from build123d import *

# Parameters (mm, degrees)
SKETCH1_R           = 16.15
BOSS_EXTRUDE1_DEPTH = 5.2
FILLET1_R           = 20
CHAMFER1_SIZE       = 1
SKETCH2_R           = 19.025242353
SKETCH2_R_2         = 14
BOSS_EXTRUDE2_DEPTH = 0.6
SKETCH4_R           = 18.71529055
SKETCH4_R_2         = 14
BOSS_EXTRUDE3_DEPTH = 1
CHAMFER2_SIZE       = 1


with BuildPart() as part:
    # Sketch1 → Boss-Extrude1 (new body)
    with BuildSketch(Plane(origin=(0, 0, 0), x_dir=(1, 0, 0), z_dir=(0, 1, 0))):
        with BuildLine():
            Line((50.6952797, -21), (63.625, -21))
            ThreePointArc((63.625, -21), (84.625, 0), (63.625, 21))
            Line((63.625, 21), (50.6952797, 21))
            ThreePointArc((50.6952797, 21), (44.646090821, 13.026866227), (35.106613419, 10))
            Line((35.106613419, 10), (-35.106613419, 10))
            ThreePointArc((-35.106613419, 10), (-44.646090821, 13.026866227), (-50.6952797, 21))
            Line((-50.6952797, 21), (-63.625, 21))
            ThreePointArc((-63.625, 21), (-84.625, 0), (-63.625, -21))
            Line((-63.625, -21), (-50.6952797, -21))
            ThreePointArc((-50.6952797, -21), (-44.646090821, -13.026866227), (-35.106613419, -10))
            Line((-35.106613419, -10), (35.106613419, -10))
            ThreePointArc((35.106613419, -10), (44.646090821, -13.026866227), (50.6952797, -21))
        make_face()
        with Locations((-63.625, 0)):
            Circle(SKETCH1_R, mode=Mode.SUBTRACT)
        with Locations((63.625, 0)):
            Circle(SKETCH1_R, mode=Mode.SUBTRACT)
    extrude(amount=BOSS_EXTRUDE1_DEPTH)

    # Fillet1
    fillet1_edges = [part.edges().sort_by_distance(p)[0] for p in [
        (-50.6952797, 2.6, 21),
        (-50.6952797, 2.6, -21),
        (50.6952797, 2.6, -21),
        (50.6952797, 2.6, 21),
    ]]
    fillet(fillet1_edges, radius=FILLET1_R)

    # Chamfer1
    chamfer1_edges = [part.edges().sort_by_distance(p)[0] for p in [
        (62.433003391, 5.2, 21),
        (84.625, 5.2, 0),
        (62.433003391, 5.2, -21),
        (41.52534742, 5.2, -11.295776268),
        (0, 5.2, -10),
        (41.52534742, 5.2, 11.295776268),
        (-41.52534742, 5.2, -11.295776268),
        (-62.433003391, 5.2, -21),
        (-62.433003391, 5.2, 21),
        (-53.482236449, 5.2, 19.433705079),
        (-53.482236449, 5.2, -19.433705079),
        (-84.625, 5.2, 0),
        (53.482236449, 5.2, -19.433705079),
        (53.482236449, 5.2, 19.433705079),
        (-41.52534742, 5.2, 11.295776268),
        (0, 5.2, 10),
        (47.475, 5.2, 0),
    ]]
    chamfer(chamfer1_edges, length=CHAMFER1_SIZE)

    # Sketch2 → Boss-Extrude2 (add)
    with BuildSketch(Plane.XZ):
        with Locations((63.625, 0)):
            Circle(SKETCH2_R)
        with Locations((63.625, 0)):
            Circle(SKETCH2_R_2, mode=Mode.SUBTRACT)
    extrude(amount=-BOSS_EXTRUDE2_DEPTH)

    # Sketch4 → Boss-Extrude3 (add)
    with BuildSketch(Plane(origin=(0, 5.2, 0), x_dir=(1, 0, 0), z_dir=(0, 1, 0))):
        with Locations((-63.625, 0)):
            Circle(SKETCH4_R)
        with Locations((-63.625, 0)):
            Circle(SKETCH4_R_2, mode=Mode.SUBTRACT)
    extrude(amount=-BOSS_EXTRUDE3_DEPTH)

    # Chamfer2
    chamfer2_edges = [part.edges().sort_by_distance(p)[0] for p in [
        (-79.775, 0, 0),
    ]]
    chamfer(chamfer2_edges, length=CHAMFER2_SIZE)


solid = part.part
Geometry: final body of the model. Coordinates: model frame, mm. A direction names the side the tool comes from. Give positions to 0.01 mm unless a question says otherwise; leave off trailing zeros. Write each loop counter-clockwise with the first axis right and the second up, starting at its lowest first coordinate (ties: lowest second). Pieces come first, ordered by that corner, then holes.
(1) Mould query, pull axis Z, two halves, no side actions, for faces 1 (the conical face through (-83.78, 5.04, -0.44)), 2 (the cylindrical face through (47.49, 2.37, -0.71)), 3 (the flat face through (0, 2, -10)), 4 (the flat face through (-76, 4.2, -7)). Classes: released by +Z, released by -Z, zero draft, split by the parting line, or undercut.
(2) Access query for faces 5 (the cylindrical face through (-53.4, 2.1, -19.4)), 6 (the cylindrical face through (-79.76, 2.58, -0.71)), 7 (the cylindrical face through (-53.4, 2.1, 19.4)), 8 (the flat face through (63.5, 0.6, 14.4)), 9 (the conical face through (83.78, 5.04, 0.44)). Directions: +Z, -Z, +X, -X, +Y, -Y. A direction counts if a zero-diameter tool reaches every point of the face in a straight line with its end or side. Return the directions, or none.
(3) Cut plane B-B, the plane y = 2.15. Give the number of separate pieces and of enclosed holes in the cut face, then the cut area to 3 significant figures.
(4) Ray query, line 1 (X direction, y = 1.35, z = 0) (3 decimals); line 2 (X direction, y = 3, z = 15); line 3 (X direction, y = 4.55, z = 0) (3 decimals). Return the intervals inside material, ascending.
(5) Cut plane A-A, the plane z = 0. Return loops of the section in (x, y) (3 decimals), then the cut area to 3 significant figures.
Values follow:
1. face 1: split by the parting line
1. face 2: undercut
1. face 3: released by -Z
1. face 4: undercut
2. face 5: -Z, +Y, -Y
2. face 6: -Y
2. face 7: +Z, +Y, -Y
2. face 8: +Y
2. face 9: +X, +Y
3. separate pieces: 1
3. enclosed holes: 2
3. area: 2,990 mm2
4. line 1: x = -84.625 to -79.775, -47.475 to 47.475, 79.775 to 84.625
4. line 2: x = -78.32 to -69.61, -57.64 to -46.96, 46.96 to 57.64, 69.61 to 78.32
4. line 3: x = -84.275 to -77.625, -49.625 to 47.125, 80.125 to 84.275
5. outline: (-84.625, 0) - (-80.775, 0) - (-79.775, 1) - (-79.775, 4.2) - (-77.625, 4.2) - (-77.625, 5.2) - (-83.625, 5.2) - (-84.625, 4.2) - close; (-49.625, 4.2) - (-47.475, 4.2) - (-47.475, 1) - (-46.475, 0) - (49.625, 0) - (49.625, 0.6) - (47.475, 0.6) - (47.475, 4.2) - (46.475, 5.2) - (-49.625, 5.2) - close; (77.625, 0) - (84.625, 0) - (84.625, 4.2) - (83.625, 5.2) - (80.775, 5.2) - (79.775, 4.2) - (79.775, 0.6) - (77.625, 0.6) - close
5. area: 548 mm2
